Source: CAD feature listing. Evaluate the final solid. Frame: model axes, mm. A direction names the side the tool comes from. Coordinates: 2 decimals unless noted, no trailing zeros. Loops run counter-clockwise (first coordinate to the right, second up) from the corner with the lowest first, then second, coordinate; pieces in that order, holes last. Notation, with made-up numbers: M 56,28.5 L 68,28.5 A26 cw 68,57.5 Z; hole C -36.75,11.25 d7. An arc over 180 degrees is marked long. One line per question, with ' | ' between items. Start each with the question number.
1. Pin query (flat end, axial travel): P1, Ø0.6, axis at x = -0.5, z = -0.5, coming from the -Y side; P2, Ø6, axis at x = 5.5, y = 12, coming from the -Z side; P3, Ø4, axis at x = 0.5, y = 24, coming from the -Z side. Return the tip coordinate at first contact, or that it passes through.
2. Access query for faces 4 (the flat face through (10, 0, 0)), 5 (the cylindrical face through (-1, 9, 0)). Directions: +Z, -Z, +X, -X, +Y, -Y. A direction counts if a zero-diameter tool reaches every point of the face in a straight line with its end or side. Return the directions, or none.
3. Ray query, probe 1 along Y at (x, z) = (9, -0.6); probe 2 along Y at (x, z) = (7, -0.1); probe 3 along X at (y, z) = (26.5, 0.05). Return the intervals inside material, ascending.
4. Section query A-A, the plane z = 0. Output: boundary loops of the cut face in (x, y), and give its area (3 significant figures).
5. Mould query, pull axis Y, two halves, no side actions, for faces 1 (the cylindrical face through (-1, 22, 0)), 2 (the cylindrical face through (6, -1, 0)), 3 (the cylindrical face through (0.63, 16.01, 0.49)). Classes: pulls with the +Y half, pulls with the -Y half, needs draft (parallel to the pull), parting line crosses it, or undercut.
6. Section query B-B, the plane y = 13. Output: boundary loops of the cut face in (x, z), and give its area (3 significant figures).
```python
from build123d import *

# Parameters (mm, degrees)
SKETCH2_R = 1
SKETCH3_W = 0.2
SKETCH3_H = 1


with BuildPart() as part:
    # Sweep1: sweep along a path in Sketch1
    with BuildLine(Plane.XY) as sweep1_path:
        Line((0, 30), (0, 2))
        ThreePointArc((0, 2), (0.585786438, 0.585786438), (2, 0))
        Line((2, 0), (10, 0))
    # Sketch2 → Sweep1 (sweep)
    with BuildSketch(Plane(origin=(10, 0, 0), x_dir=(0, 0, -1), z_dir=(1, 0, 0))):
        Circle(SKETCH2_R)
    sweep(path=sweep1_path.line)

    # Sketch3 → Cut-Revolve1 (revolve, cut)
    with BuildSketch(Plane.XY):
        Polygon((-0.3, 30), (-1, 28), (-1, 30), align=None)
        with Locations((-0.9, 16)):
            Rectangle(SKETCH3_W, SKETCH3_H)
    revolve(axis=Axis((0, 30, 0), (0, -1, 0)), mode=Mode.SUBTRACT)


solid = part.part
```
Taken from the geometry:
1) P1: y = 0.1 | P2: through | P3: z = -1
2) face 4: +Z, -Z, +X, +Y, -Y | face 5: +Y
3) probe 1: -0.8 to 0.8 | probe 2: -0.99 to 0.99 | probe 3: -1 to 1
4) outline: M -1,2 A3 ccw 2,-1 L 10,-1 L 10,1 L 2,1 A1 cw 1,2 L 1,15.5 L 0.8,15.5 L 0.8,16.5 L 1,16.5 L 1,28 L 0.3,30 L -0.3,30 L -1,28 L -1,16.5 L -0.8,16.5 L -0.8,15.5 L -1,15.5 Z | area: 76.5 mm^2
5) face 1: needs draft | face 2: parting line crosses it | face 3: undercut
6) outline: C 0,0 d2 | area: 3.14 mm^2
